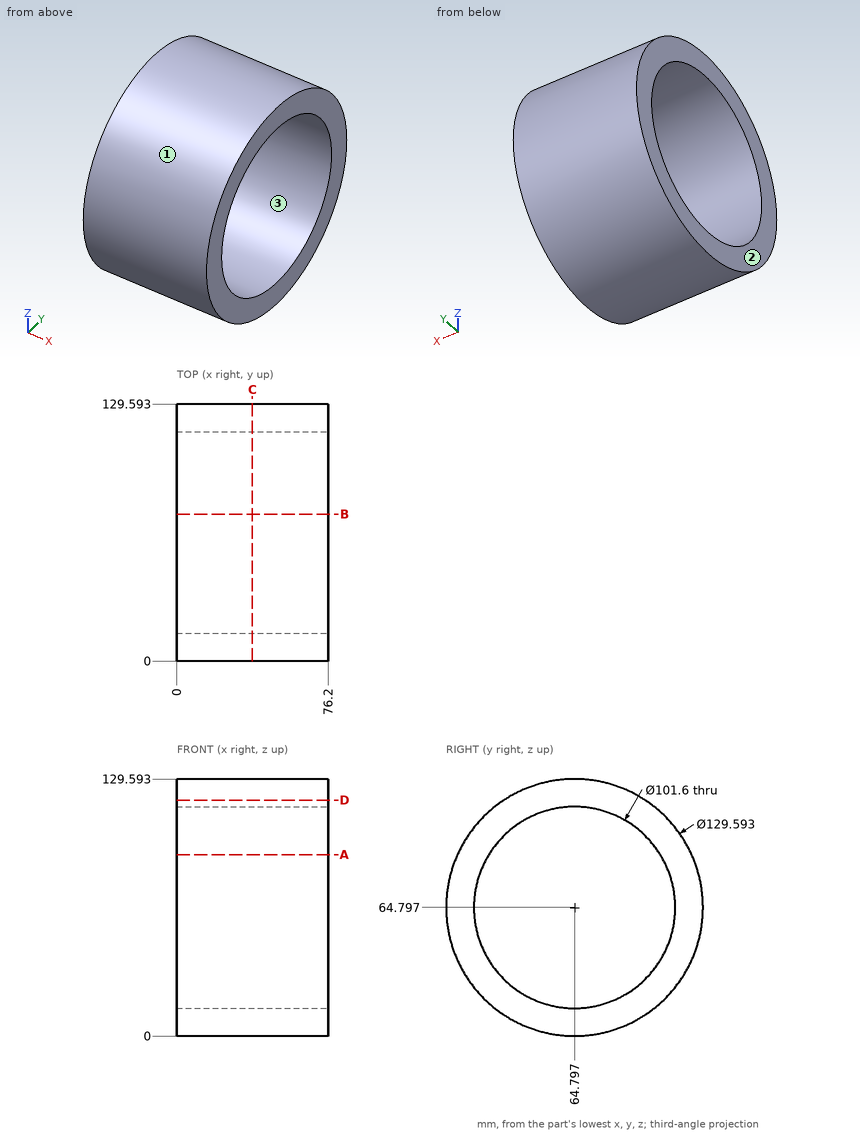
Input: dimensioned drawing with shaded views. Units: mm. Origin: part minimum x, y, z. Give positions to 0.01 mm unless a question says otherwise; leave off trailing zeros. Write each loop counter-clockwise with the first axis right and the second up, starting at its lowest first coordinate (ties: lowest second). Pieces come first, ordered by that corner, then holes.
Q1. Section B-B, the plane y = 74. Output: boundary loops of the cut face in (x, z).
Q2. Section C-C, the plane x = 38. Output: boundary loops of the cut face in (y, z), plus the area to 3 significant figures.
Q3. Section D-D, the plane z = 119. Output: boundary loops of the cut face in (x, y).
Q4. Section A-A, the plane z = 91.5. Output: boundary loops of the cut face in (x, y) (1 decimal), plus the area to 3 significant figures.
Q5. First-contact query: P1, Ø12, axis at x = 19, z = 72, coming from the -Y side; P2, Ø6, axis at x = 42, y = 74.5, coming from the +Z side; P3, Ø2, axis at y = 15.5, z = 68, coming from the +X side; P4, Ø3, axis at x = 44.5, z = 94, coming from the +Y side. Flat tips, straight axial feed; report the tip coordinate or a pass-through.
Q6. Pull-direction query (Y, two-part tool) for the marked faces 1, 2 and 3; classes: pulls with the +Y half, pulls with the -Y half, needs draft (parallel to the pull), parting line crosses it, or undercut.
Q7. Material intervals for probe 1 along Z at (x, y) = (36, 66); probe 2 along Y at (x, z) = (34.5, 47.5); probe 3 along Y at (x, z) = (41, 64) (1 decimal), sorted ascending.
Filled in:
1. outline: (0, 0.66) - (76.2, 0.66) - (76.2, 14.84) - (0, 14.84) - close; (0, 114.76) - (76.2, 114.76) - (76.2, 128.94) - (0, 128.94) - close
2. outline: circle Ø129.59 at (64.8, 64.8); hole circle Ø101.6 at (64.8, 64.8)
2. area: 5,080 mm2
3. outline: (0, 29.29) - (76.2, 29.29) - (76.2, 100.3) - (0, 100.3) - close
4. outline: (0, 5.8) - (76.2, 5.8) - (76.2, 21.6) - (0, 21.6) - close; (0, 108) - (76.2, 108) - (76.2, 123.8) - (0, 123.8) - close
4. area: 2,410 mm2
5. P1: stops at y = 0.01
5. P2: stops at z = 129.25
5. P3: passes through
5. P4: stops at y = 123.37
6. face 1: parting line crosses it
6. face 2: needs draft
6. face 3: undercut
7. probe 1: z = 0.01 to 14.01, 115.58 to 129.58
7. probe 2: y = 2.35 to 17.03, 112.56 to 127.24
7. probe 3: y = 0 to 14, 115.6 to 129.6
